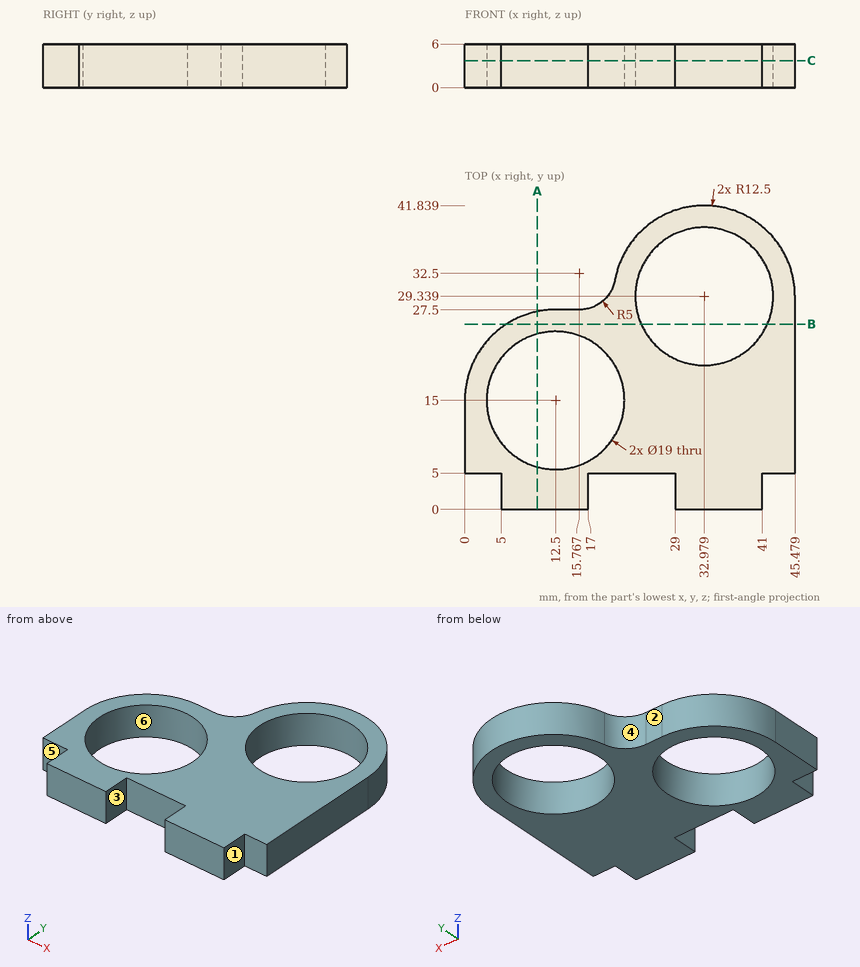
Here's the drawing with two shaded views (mm, measured from the low corner). I have some questions. A direction names the side the tool comes from. Coordinates: 2 decimals unless noted, no trailing zeros. Write each loop counter-clockwise with the first axis right and the second up, starting at its lowest first coordinate (ties: lowest second). Pieces come first, ordered by that corner, then holes. Notation, with made-up numbers: (-32, -8.5) -> (9, -8.5) arc R6 cw to (9, -0.5) -> close; hole circle Ø6 at (-37.75, 22.25). An arc over 180 degrees is marked (long way). Use a Markdown table: item, result. Add a question column.
(1) I'm going to push flat-ended pins straight in: P1, Ø4, axis at x = 32, y = 22, coming from the +Z side; P2, Ø1.5, axis at x = 1.5, z = 3.5, coming from the -Y side; P3, Ø1.5, axis at x = 34, z = 5, coming from the +Y side; P4, Ø2.5, axis at y = 2.5, z = 2, coming from the -X side. Where does each tip first touch, or does it pass through?
(2) If we section it at A-A, the plane x = 10: Write out the boundary of the cut face in (y, z) (1 decimal).
(3) We'd pull the mould along X, two halves only. Please class the marked faces 4, 5 and 6: +X half, -X half, draft (parallel to the pull), parting line (faces both ways), or undercut.
(4) For the marked faces 1, 2 and 3, which set-ups out of +Z, -Z, +X, -X, +Y, -Y let a thin tool reach every point of the face, with its end or its side?
(5) If we section it at B-B, the plane y = 25.5: Write out the boundary of the cut face in (x, z).
(6) If we section it at C-C, the plane z = 3.7: Write out the boundary of the cut face in (x, y) (1 decimal).
(7) Please list where these lines run through material, in increasing order: line 1 (X direction, y = 4, z = 4.15); line 2 (X direction, y = 22, z = 3.45) (1 decimal); line 3 (X direction, y = 21.5, z = 5) (1 decimal).
Outcome:
| question | item | result |
|---|---|---|
| 1 | P1 | passes through |
| 1 | P2 | stops at y = 5 |
| 1 | P3 | stops at y = 41.84 |
| 1 | P4 | stops at x = 5 |
| 2 | outline | (0, 0) -> (5.8, 0) -> (5.8, 6) -> (0, 6) -> close; (24.2, 0) -> (27.2, 0) -> (27.2, 6) -> (24.2, 6) -> close |
| 3 | face 4 | -X half |
| 3 | face 5 | draft |
| 3 | face 6 | undercut |
| 4 | face 1 | +Z, -Z, +X, -Y |
| 4 | face 2 | +Z, -Z, -X, +Y |
| 4 | face 3 | +Z, -Z, -Y |
| 5 | outline | (5.72, 0) -> (24.29, 0) -> (24.29, 6) -> (5.72, 6) -> close; (41.67, 0) -> (45.48, 0) -> (45.48, 6) -> (41.67, 6) -> close |
| 6 | outline | (0, 5) -> (5, 5) -> (5, 0) -> (17, 0) -> (17, 5) -> (29, 5) -> (29, 0) -> (41, 0) -> (41, 5) -> (45.5, 5) -> (45.5, 29.3) arc R12.5 ccw to (20.7, 31.6) arc R5 cw to (15.8, 27.5) -> (12.5, 27.5) arc R12.5 ccw to (0, 15) -> close; hole circle Ø19 at (12.5, 15); hole circle Ø19 at (33, 29.3) |
| 7 | line 1 | x = 5 to 17, 29 to 41 |
| 7 | line 2 | x = 2.1 to 6.1, 18.9 to 26.9, 39 to 45.5 |
| 7 | line 3 | x = 1.8 to 5.6, 19.4 to 27.6, 38.3 to 45.5 |
